Part model, mm, in its own coordinate system. A direction names the side the tool comes from. Give positions to 0.01 mm unless a question says otherwise; leave off trailing zeros. Order: outer loops, then holes, each group sorted by start corner. A loop starts at its lowest first (then second) coordinate and runs counter-clockwise, first axis right, second up. Notation, with made-up numbers: M 2.25,18 L 34.25,18 A20 cw 34.25,25 Z; hole C 77,30.25 d3. An arc over 180 degrees is marked long. Write each question's results on one line, items separated by ' | '. Start each with the question number.
from build123d import *

# Parameters (mm, degrees)
BOSS_EXTRUDE1_DEPTH = 93.98
SKETCH2_R           = 5.499261314
SKETCH2_R_2         = 4.7625
CUT_EXTRUDE1_DEPTH  = 9.0424


with BuildPart() as part:
    # Sketch1 → Boss-Extrude1 (new body)
    with BuildSketch(Plane(origin=(0, 0, 0), x_dir=(0, 0, -1), z_dir=(1, 0, 0))):
        Polygon((-5.499261314, 0), (-2.749630657, -4.7625), (2.749630657, -4.7625), (5.499261314, 0), (2.749630657, 4.7625), (-2.749630657, 4.7625), align=None)
    extrude(amount=BOSS_EXTRUDE1_DEPTH)

    # Sketch2 → Cut-Extrude1 (cut)
    with BuildSketch(Plane(origin=(93.98, 0, 0), x_dir=(0, 0, -1), z_dir=(1, 0, 0))):
        Circle(SKETCH2_R)
        Circle(SKETCH2_R_2, mode=Mode.SUBTRACT)
    extrude(amount=-CUT_EXTRUDE1_DEPTH, mode=Mode.SUBTRACT)


solid = part.part
(1) Drop a flat-ended pin along its axis: P1, Ø2, axis at y = 1, z = 2.5, coming from the -X side. Give the stop position or say it passes through.
(2) Tool access for faces 1 (the flat face through (84.938, 4, -3)), 2 (the flat face through (84.938, -4.3, 2.4)), 3 (the flat face through (84.938, 4.3, 2.4)), 4 (the flat face through (84.938, -4, -3)): list every direction of +Z, -Z, +X, -X, +Y, -Y with a clear straight run to the whole face (end or side of a thin tool).
(3) Saw through at A-A on x = 30. Give the cut face in (y, z), plus the area to 3 significant figures.
(4) Saw through at B-B on y = 1.5. Give the cut face in (x, z), plus the area to 3 significant figures.
(5) Probe L1, parallel to Y at x = 34.5, z = -5; L2, parallel to Z at x = 34.5, y = 2.25; L3, parallel to Y at x = 58.5, z = -3. List the from-to ranges inside material, lowest first.
Taken from the geometry:
1) P1: stops at x = 0
2) face 1: -Z, +X, +Y | face 2: +Z, +X, -Y | face 3: +Z, +X, +Y | face 4: -Z, +X, -Y
3) outline: M -4.76,-2.75 L 0,-5.5 L 4.76,-2.75 L 4.76,2.75 L 0,5.5 L -4.76,2.75 Z | area: 78.6 mm²
4) outline: M 0,-4.63 L 84.94,-4.63 L 84.94,-4.52 L 93.98,-4.52 L 93.98,4.52 L 84.94,4.52 L 84.94,4.63 L 0,4.63 Z | area: 869 mm²
5) L1: y = -0.86 to 0.86 | L2: z = -4.2 to 4.2 | L3: y = -4.33 to 4.33
